from build123d import *

# Parameters (mm, degrees)
CROQUIS3_W                 = 50
CROQUIS3_H                 = 42
SALIENTE_EXTRUIR7_DEPTH    = 8
CORTAR_EXTRUIR2_DEPTH      = 8
CORTAR_EXTRUIR2_DEPTH_BACK = 8
CROQUIS3_13_W              = 46.428571428
CROQUIS3_13_H              = 39
REDONDEO3_R                = 21
CROQUIS7_W                 = 3.39365255
CROQUIS7_H                 = 46.015277421
CORTAR_EXTRUIR3_DEPTH      = 8


with BuildPart() as part:
    # Croquis3 → Saliente-Extruir7 (new body)
    with BuildSketch(Plane(origin=(0, 0, 0), x_dir=(1, 0, 0), z_dir=(0, 1, 0))):
        with Locations((25, 21)):
            Rectangle(CROQUIS3_W, CROQUIS3_H)
    extrude(amount=SALIENTE_EXTRUIR7_DEPTH)

    # Croquis3<13> → Cortar-Extruir2 (cut, two sides: drawn at the far end of the back side and taken through both)
    with BuildSketch(Plane(origin=(0, 0, 0), x_dir=(1, 0, 0), z_dir=(0, 1, 0)).offset(-CORTAR_EXTRUIR2_DEPTH_BACK)):
        with Locations((25, 21)):
            Rectangle(CROQUIS3_13_W, CROQUIS3_13_H)
    extrude(amount=CORTAR_EXTRUIR2_DEPTH + CORTAR_EXTRUIR2_DEPTH_BACK, mode=Mode.SUBTRACT)

    # Redondeo3
    # the kernel refuses this fillet: 21 mm, written as the material it adds along each edge
    with BuildSketch(Plane(origin=(1.785714286, 0, -1.5), x_dir=(0, 0, -1), z_dir=(0, 1, 0)), Plane(origin=(1.785714286, 0, -40.5), x_dir=(1, 0, 0), z_dir=(0, 1, 0))) as redondeo3_piece_1:
        with BuildLine():
            CenterArc((REDONDEO3_R, -REDONDEO3_R), REDONDEO3_R, 90, 90)
            Line((0, -REDONDEO3_R), (0, 0))
            Line((0, 0), (REDONDEO3_R, 0))
        make_face()
    extrude(amount=8)
    # the kernel refuses this fillet: 21 mm, written as the material it takes off along each edge
    with BuildSketch(Plane(origin=(0, -52.5, 0), x_dir=(1, 0, 0), z_dir=(0, 1, 0)), Plane(origin=(0, -52.5, -42), x_dir=(0, 0, 1), z_dir=(0, 1, 0))) as redondeo3_2_piece_1:
        with BuildLine():
            CenterArc((REDONDEO3_R, REDONDEO3_R), REDONDEO3_R, 180, 90)
            Line((0, REDONDEO3_R), (0, 0))
            Line((0, 0), (REDONDEO3_R, 0))
        make_face()
    extrude(amount=113, mode=Mode.SUBTRACT)

    # Croquis7 → Cortar-Extruir3 (cut)
    with BuildSketch(Plane(origin=(0, 8, 0), x_dir=(1, 0, 0), z_dir=(0, 1, 0))):
        with Locations((49.446476979, 20.219134687)):
            Rectangle(CROQUIS7_W, CROQUIS7_H)
    extrude(amount=-CORTAR_EXTRUIR3_DEPTH, mode=Mode.SUBTRACT)


solid = part.part
Read the model definition and answer for the solid it produces. Units are mm, in the model's axes. A direction names the side the tool comes from. Coordinates: 2 decimals unless noted, no trailing zeros. Write each loop counter-clockwise with the first axis right and the second up, starting at its lowest first coordinate (ties: lowest second). Pieces come first, ordered by that corner, then holes. Notation, with made-up numbers: M 71.25,68.5 L 82.25,68.5 A29 ccw 82.25,103.5 Z; hole C 64,19 d2. An arc over 180 degrees is marked long. Use a Markdown table: item, result.
Q1. The part is cut by section C-C, the plane x = 18. Write down the section's boundary in (y, z).
Answer block:
| item | result |
|---|---|
| outline | M 0,-41.78 L 8,-41.78 L 8,-39.95 L 0,-39.95 Z; M 0,-2.05 L 8,-2.05 L 8,-0.22 L 0,-0.22 Z |
Q2. Straight lines are drawn through the part: L1, parallel to Z at x = 29.5, y = 1.25; L2, parallel to X at y = 6.5, z = -21; L3, parallel to Z at x = 20, y = 3. For each, find the intervals that lie inside material, in ascending order. Write a range as [from, to].
Answer block:
| item | result |
|---|---|
| L1 | z = [-42, -40.5], [-1.5, 0] |
| L2 | x = [0, 1.84] |
| L3 | z = [-41.98, -40.31], [-1.69, -0.02] |
Q3. The part is cut by section B-B, the plane y = 2.5. Write down the section's boundary in (x, z), then the cut area to 3 significant figures.
Answer block:
| item | result |
|---|---|
| outline | M 1.84,-21 A21 cw 22.79,-1.5 L 47.75,-1.5 L 47.75,0 L 21,0 A21 ccw 21,-42 L 47.75,-42 L 47.75,-40.5 L 22.79,-40.5 A21 cw Z |
| area | 213 mm2 |
Q4. The part is cut by section A-A, the plane x = 35.5. Write down the section's boundary in (y, z).
Answer block:
| item | result |
|---|---|
| outline | M 0,-42 L 8,-42 L 8,-40.5 L 0,-40.5 Z; M 0,-1.5 L 8,-1.5 L 8,0 L 0,0 Z |
Q5. Determine the mould class of faces 1 (the face through (0, 4, -21)), 2 (the face through (35, 4, -40.5)), 3 (the face through (2.5, 0, -25.8)) for opening direction Z: released by +Z, released by -Z, zero draft, split by the parting line, or undercut.
Answer block:
| item | result |
|---|---|
| face 1 | split by the parting line |
| face 2 | undercut |
| face 3 | zero draft |
Q6. Which of the six approach directions +Z, -Z, +X, -X, +Y, -Y give full straight-line access (tool end or side, diameter ignored) to faces 4 (the face through (47.75, 4, -41)), 5 (the face through (8.316, 3.944, -7.281))?
Answer block:
| item | result |
|---|---|
| face 4 | +Z, -Z, +X, +Y, -Y |
| face 5 | +X, +Y, -Y |
Q7. The part is cut by section D-D, the plane z = -3. Write down the section's boundary in (x, y).
Answer block:
| item | result |
|---|---|
| outline | M 10.18,0 L 14.99,0 L 14.99,8 L 10.18,8 Z |
Q8. This flat-tipped pin is pushed along its axis until it touches: pin 1 Ø3 at (y, z) = (1.5, -20) entering from -X. Where does it stop, or does it pass through?
Answer block:
| item | result |
|---|---|
| pin 1 | stops at x = 0 |
